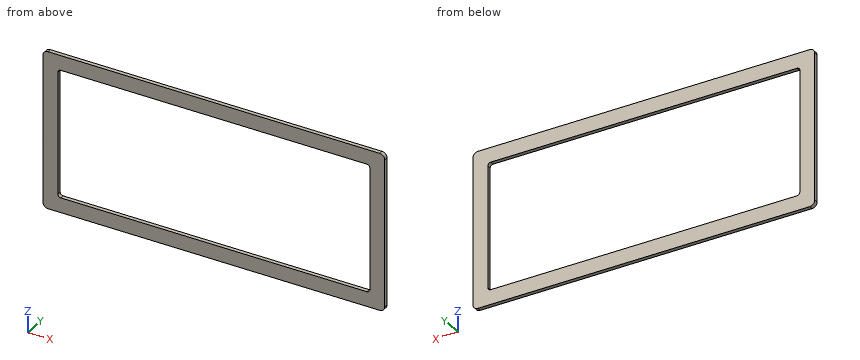
Autodesk Inventor part; units mm, degrees
ref_plane "YZ Plane" through (0, 0, 0) normal (1, 0, 0) x (0, 1, 0)
ref_plane "XZ Plane" through (0, 0, 0) normal (0, 1, 0) x (-1, 0, 0)
ref_plane "XY Plane" through (0, 0, 0) normal (0, 0, 1) x (1, 0, 0)
sketch "Sketch1" plane through (0, 0, 0) normal (0, 1, 0) x (-1, 0, 0)
  line L0 (-163.5112, 73.4938) -> (-163.5112, -76.3312)
  line L1 (-158.5112, 78.4938) -> (177.0518, 78.4938)
  arc A0 (-158.5112, 78.4938) -> (-163.5112, 73.4938) centre (-158.5112, 73.4938) ccw
  arc A1 (-163.5112, -76.3312) -> (-158.5112, -81.3312) centre (-158.5112, -76.3312) ccw
  line L2 (182.0518, -76.3312) -> (182.0518, 73.4938)
  line L3 (177.0518, -81.3312) -> (-158.5112, -81.3312)
  arc A2 (177.0518, -81.3312) -> (182.0518, -76.3312) centre (177.0518, -76.3312) ccw
  arc A3 (182.0518, 73.4938) -> (177.0518, 78.4938) centre (177.0518, 73.4938) ccw
  line L4 (-145.5232, 63.4943) -> (164.0397, 63.4943)
  line L5 (-148.5112, 60.4941) -> (-148.5112, -63.3312)
  line L6 (167.0517, 60.4941) -> (167.0517, -63.3312)
  line L7 (-145.5112, -66.3312) -> (164.0517, -66.3312)
  arc A4 (-145.5112, 63.4943) -> (-148.5112, 60.4648) centre (-145.5112, 60.4941) ccw
  arc A5 (167.0517, 60.4941) -> (164.0397, 63.4943) centre (164.1459, 60.5889) ccw
  arc A6 (164.0517, -66.3312) -> (167.0517, -63.3312) centre (164.0517, -63.3312) ccw
  arc A7 (-148.5112, -63.3312) -> (-145.5112, -66.3312) centre (-145.5112, -63.3312) ccw
  point P0 (0, 0)
extrude "Extrusion1" add sketch "Sketch1" along normal blind 4
properties part number "layer2"
Part model, mm, in its own coordinate system. Coordinates: 2 decimals unless noted, no trailing zeros. Order: outer loops, then holes, each group sorted by start corner. A loop starts at its lowest first (then second) coordinate and runs counter-clockwise, first axis right, second up. Notation, with made-up numbers: M 26,39.5 L 79,39.5 A19 cw 79,47.5 Z; hole C 77,80 d8. An arc over 180 degrees is marked long. Use a Markdown table: item, result.
(1) Probe L1, parallel to Z at x = -25, y = 1.65; L2, parallel to X at y = 3.05, z = -52; L3, parallel to X at y = 3.7, z = -66. List the from-to ranges inside material, lowest first.
A:
| item | result |
|---|---|
| L1 | z = -81.33 to -66.33, 63.49 to 78.49 |
| L2 | x = -182.05 to -167.05, 148.51 to 163.51 |
| L3 | x = -182.05 to -165.42, 146.88 to 163.51 |
(2) Cut at B-B on y = 1.2. Write the cut outline in (x, z).
A:
| item | result |
|---|---|
| outline | M -182.05,-76.33 A5 ccw -177.05,-81.33 L 158.51,-81.33 A5 ccw 163.51,-76.33 L 163.51,73.49 A5 ccw 158.51,78.49 L -177.05,78.49 A5 ccw -182.05,73.49 Z; hole M -167.05,-63.33 A3 ccw -164.05,-66.33 L 145.51,-66.33 A3 ccw 148.51,-63.33 L 148.51,60.49 A3 ccw 145.52,63.49 L -164.04,63.49 A2.91 ccw -167.05,60.49 Z |
(3) Cut at A-A on x = 11. Write the cut outline in (y, z).
A:
| item | result |
|---|---|
| outline | M 0,-81.33 L 4,-81.33 L 4,-66.33 L 0,-66.33 Z; M 0,63.49 L 4,63.49 L 4,78.49 L 0,78.49 Z |
(4) Cut at C-C on z = 9.5. Write the cut outline in (x, y), then the cut area to 3 significant figures.
A:
| item | result |
|---|---|
| outline | M -182.05,0 L -167.05,0 L -167.05,4 L -182.05,4 Z; M 148.51,0 L 163.51,0 L 163.51,4 L 148.51,4 Z |
| area | 120 mm^2 |
